Could you check a few things on this model? Use its own coordinates, in mm. Face numbers are marked on the shaded views. A direction names the side the tool comes from. Coordinates: 2 decimals unless noted, no trailing zeros. Loops run counter-clockwise (first coordinate to the right, second up) from the corner with the lowest first, then second, coordinate; pieces in that order, holes last.
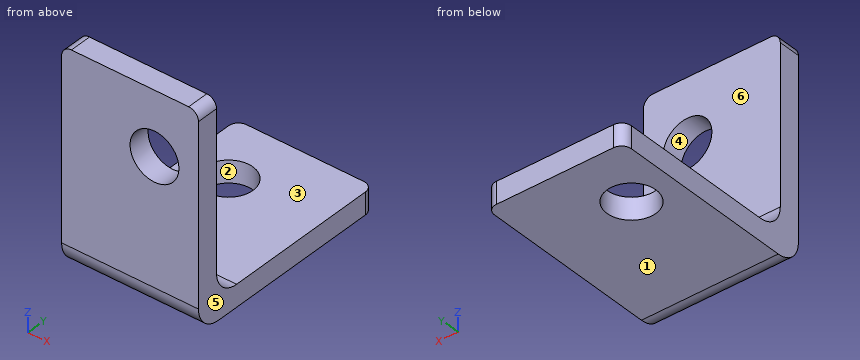
Autodesk Inventor part; units mm, degrees
ref_plane "YZ Plane" through (0, 0, 0) normal (1, 0, 0) x (0, 1, 0)
ref_plane "XZ Plane" through (0, 0, 0) normal (0, 1, 0) x (-1, 0, 0)
ref_plane "XY Plane" through (0, 0, 0) normal (0, 0, 1) x (1, 0, 0)
sketch "Sketch1" plane through (0, 0, 0) normal (1, 0, 0) x (0, 1, 0)
  line L0 (0, 0) -> (4.5, 0)
  line L1 (4.5, 0) -> (4.5, -39.16)
  line L2 (1.7807, -43.66) -> (0, -43.66)
  line L3 (0, -43.66) -> (0, 0)
  line L4 (0, -43.66) -> (43.6, -43.66)
  line L5 (43.6, -43.66) -> (43.6, -39.16)
  line L6 (43.6, -39.16) -> (4.5, -39.16)
  line L7 (0, -7.4197) -> (0, -43.66)
  dimension "d0" = 43.6
  dimension "d1" = 43.66
  dimension "d2" = 4.5
  dimension "d3" = 4.5
extrude "Extrusion1" add sketch "Sketch1" along normal blind 28
sketch "Sketch2" plane through (0, 4.5, 0) normal (0, 1, 0) x (1, 0, 0)
  circle A0 centre (19, 13) radius 5
  line L0 (28, 39.16) -> (28, 0)
  line L1 (0, 0) -> (28, 0)
  dimension "d6" = 10
  dimension "d7" = 9
  dimension "d8" = 13
sketch "Sketch3" plane through (0, 0, -43.66) normal (0, 0, -1) x (-1, 0, 0)
  circle A0 centre (-9, 30.6) radius 5
  line L0 (0, 0) -> (0, 43.6)
  line L1 (0, 43.6) -> (-28, 43.6)
  dimension "d9" = 9
  dimension "d10" = 13
  dimension "d11" = 10
extrude "Extrusion2" cut sketch "Sketch3" against normal up to next
extrude "Extrusion3" cut sketch "Sketch2" against normal up to next
fillet "Fillet1" radius 2 4 edges at (0, 43.6, -41.41) (28, 43.6, -41.41) (0, 2.25, 0) (28, 2.25, 0)
fillet "Fillet2" radius 5 2 edges at (14, 0, -43.66) (14, 4.5, -39.16)
properties part number "shin_L_bracket"
(1) We'd pull the mould along Z, two halves only. Please class the marked faces 1, 2, 3 and 4: +Z half, -Z half, draft (parallel to the pull), parting line (faces both ways), or undercut.
Answers:
face 1: -Z half
face 2: draft
face 3: +Z half
face 4: undercut
(2) Imagine slicing it at C-C, the plane y = 30.6. Write out the boundary of the cut face in (x, z), and give its area (3 significant figures).
Answers:
outline: (0, -43.66) - (4, -43.66) - (4, -39.16) - (0, -39.16) - close; (14, -43.66) - (28, -43.66) - (28, -39.16) - (14, -39.16) - close
area: 81.0 mm2
(3) Which directions (+Z, -Z, +X, -X, +Y, -Y) give clear straight access to the entire face, cutting with the end or side of a thin tool? Please do the marked faces 5 and 6.
Answers:
face 5: +Z, -Z, +X, +Y, -Y
face 6: +Z, +X, -X, +Y
(4) Imagine slicing it at D-D, the plane x = 13.25. Write out the boundary of the cut face in (y, z), and give its area (3 significant figures).
Answers:
outline: (0, -38.66) arc R5 ccw to (5, -43.66) - (27.97, -43.66) - (27.97, -39.16) - (9.5, -39.16) arc R5 cw to (4.5, -34.16) - (4.5, 0) - (0, 0) - close; (33.23, -43.66) - (43.6, -43.66) - (43.6, -39.16) - (33.23, -39.16) - close
area: 349 mm2
(5) For pin 1 (8.5 mm diameter, centred on x = 18.5, z = -19, fed in from +Y); pin 2 (3 mm diameter, centred on x = 18, y = 11, fed in from +Z), each with a flat end and sliding along its axis, tell me the tip position at first contact or that it passes through.
Answers:
pin 1: stops at y = 4.5
pin 2: stops at z = -39.16
(6) I need wall thicknesses on probe 1 along X at (y, z) = (2.45, -13); probe 2 along Y at (x, z) = (10.75, -3.5); probe 3 along Z at (x, y) = (23.75, 39). Which ranges of each line are inside material? Lowest first, please.
Answers:
probe 1: x = 0 to 14, 24 to 28
probe 2: y = 0 to 4.5
probe 3: z = -43.66 to -39.16
(7) Imagine slicing it at A-A, the plane x = 9. Write out the boundary of the cut face in (y, z).
Answers:
outline: (0, -38.66) arc R5 ccw to (5, -43.66) - (25.6, -43.66) - (25.6, -39.16) - (9.5, -39.16) arc R5 cw to (4.5, -34.16) - (4.5, 0) - (0, 0) - close; (35.6, -43.66) - (43.6, -43.66) - (43.6, -39.16) - (35.6, -39.16) - close
(8) Imagine slicing it at B-B, the plane z = -13. Write out the boundary of the cut face in (x, y).
Answers:
outline: (0, 0) - (14, 0) - (14, 4.5) - (0, 4.5) - close; (24, 0) - (28, 0) - (28, 4.5) - (24, 4.5) - close
